```python
from build123d import *

# Parameters (mm, degrees)
F9_D            = 6.35
F9_COPIES_COUNT = 12


# Not quite as in the source:
# - a pattern or mirror of a feature is missing from the dataset's text; its kind, count and spacing are read off the source's solid


with BuildPart() as f1:
    # F0 (on Front) → F1 (revolve)
    with BuildSketch(Plane.XZ):
        with BuildLine():
            ThreePointArc((0, 127), (89.8025612107, 89.8025612107), (127, 0))
            Line((127, 0), (127, -6.35))
            Line((127, -6.35), (133.35, -6.35))
            Line((133.35, -6.35), (133.35, 0))
            Line((133.35, 0), (171.45, 0))
            Line((171.45, 0), (171.45, 6.35))
            Line((171.45, 6.35), (133.1987237176, 6.35))
            ThreePointArc((133.1987237176, 6.35), (92.0202423383, 96.5116443752), (0, 133.35))
            Line((0, 133.35), (0, 127))
        make_face()
    revolve(axis=Axis((0, 0, 13.3139304817), (0, 0, 1)))

    # F4 (on Front) → F5 (revolve, cut)
    with BuildSketch(Plane.XZ):
        with BuildLine():
            ThreePointArc((89.8025612107, 89.8025612107), (94.1857207861, 85.1941899427), (98.3326763457, 80.3721641036))
            Line((98.3326763457, 80.3721641036), (100.7753060106, 82.8147937685))
            Line((100.7753060106, 82.8147937685), (103.0203700409, 80.5697297382))
            Line((103.0203700409, 80.5697297382), (110.3632345412, 87.9125942385))
            Line((110.3632345412, 87.9125942385), (94.2926892712, 94.2926892712))
            Line((94.2926892712, 94.2926892712), (89.8025612107, 89.8025612107))
        make_face()
    f5 = revolve(axis=Axis((92.047625241, 0, 92.047625241), (0.7071067812, 0, 0.7071067812)), mode=Mode.SUBTRACT)

    # F5_copies: F5 across plane
    add(f5.mirror(Plane(origin=(0, 0, 0), x_dir=(0, 0, -1), z_dir=(-1, 0, 0))), mode=Mode.SUBTRACT)

    # F6 (on Front) → F7 (revolve, cut)
    with BuildSketch(Plane.XZ):
        with BuildLine():
            ThreePointArc((-7.9375, 126.7517104175), (-3.9706911856, 126.9379124277), (0, 127))
            Line((0, 127), (0, 133.35))
            ThreePointArc((0, 133.35), (-3.9705104321, 133.2908757076), (-7.9375, 133.1135552592))
            Line((-7.9375, 133.1135552592), (-7.9375, 126.7517104175))
        make_face()
    revolve(axis=Axis((0, 0, 130.175), (0, 0, 1)), mode=Mode.SUBTRACT)

    # F9 (through all)
    with Locations(Plane.XY.offset(6.35)):
        with Locations((0, -152.3243618588)):
            f9 = Hole(F9_D / 2)

    # F9_copies: F9 ×12 about axis
    f9_copies_axis = Axis((0, 0, 0), (0, 0, 1))
    for i in range(1, F9_COPIES_COUNT):
        add(f9.rotate(f9_copies_axis, i * 360 / F9_COPIES_COUNT), mode=Mode.SUBTRACT)


solid = f1.part
```
The model under review builds one solid part; all positions refer to its coordinate system, in mm. A direction names the side the tool comes from. Round coordinates to 2 decimals unless told otherwise and drop trailing zeros. Write each loop counter-clockwise with the first axis right and the second up, starting at its lowest first coordinate (ties: lowest second). Pieces come first, ordered by that corner, then holes. Notation, with made-up numbers: M 73,-21 L 98,-21 A34 ccw 98,17 Z; hole C -16.5,66 d9. An arc over 180 degrees is marked long. Use CSV: the item, a comma, the result in double quotes. Start each with the question number.
(1) Clearance check with flat-ended pins moving along their axes: P1, Ø1, axis at y = -56.5, z = 76, coming from the +X side; P2, Ø4, axis at y = -14, z = 88.5, coming from the -X side; P3, Ø7.5, axis at x = 131.92, y = -76.16, coming from the -Z side. State where each tip first meets the part, or that it passes through.
(2) We need section C-C, the plane z = 60.5. State the section outline as (x, y) points, then the cut area to 3 significant figures.
(3) We need section B-B, the plane x = 41.5. State the section outline as (y, z) points.
(4) For line 1 along X through (y, z) = (-133, 3.5); line 2 along Z through (x, y) = (-137, 76.5); line 3 along X through (y, z) = (18, 108.5), list the stretches that pass through material, from the lowest coordinate up.
(5) Tool access review of faces 4 (the face through (91.85, 13.01, 91.74)), 5 (the face through (92.17, 144.567, 3.219)), 6 (the face through (-88, -101, 0)): name each direction out of +Z, -Z, +X, -X, +Y, -Y from which nothing blocks a thin tool from reaching the whole face with its end or side.
(6) The part is to be moulded in two halves that separate along Z. For faces 1 (the face through (98.886, -4.864, 82.295)), 2 (the face through (-91.85, 13.01, 91.74)), 3 (the face through (88, -101, 6.35)), say which applies: +Z half, -Z half, draft (parallel to the pull), parting line (faces both ways), or undercut.
Findings:
1,P1,"x = 94.38"
1,P2,"x = -100.54"
1,P3,"z = 0"
2,outline,"C 0,0 d237.67; hole C 0,0 d223.33"
2,area,"5,190 mm^2"
3,outline,"M -166.35,0 L -126.73,0 L -126.73,-6.35 L -120.03,-6.35 L -120.03,0 A120.03 cw 120.03,0 L 120.03,-6.35 L 126.73,-6.35 L 126.73,0 L 166.35,0 L 166.35,6.35 L 126.57,6.35 A126.73 ccw -126.57,6.35 L -166.35,6.35 Z"
4,line 1,"-108.19 to -79.15, -73.18 to 73.18, 79.15 to 108.19"
4,line 2,"0 to 6.35"
4,line 3,"-75.41 to -63.5, 63.5 to 75.41"
5,face 4,"none"
5,face 5,"+Z, -Z"
5,face 6,"-Z"
6,face 1,"parting line"
6,face 2,"undercut"
6,face 3,"+Z half"
